from build123d import *

# Parameters (mm, degrees)
F1_DEPTH  = 75
F3_DEPTH  = 4
F5_W      = 61.9195103645
F5_H      = 37.6517623663
F6_DEPTH  = 17
F7_DEPTH  = 44
F9_D      = 7
F9_DEPTH  = 15
F9_TIP    = 2.1030121666
F10_R     = 3.3275648112
F10_R_2   = 1.7
F11_DEPTH = 2
F12_DEPTH = 25.4


with BuildPart() as f1:
    # F0 (on Right) → F1 (new body)
    with BuildSketch(Plane.YZ):
        with BuildLine():
            add(Edge.make_bspline(
                [(-17.7810950981, -27.3124240728), (-18.19174778, -28.0218574236), (-18.6022967338, -28.732065323), (-19.0125334596, -29.4428684699)],
                knots=[0.9798659686, 0.9798659686, 0.9798659686, 0.9798659686, 1, 1, 1, 1], degree=3))
            ThreePointArc((-17.7810950981, -27.3124240728), (-18.4276280065, -28.3598353366), (-19.0125334596, -29.4428684699))
        make_face()
        with BuildLine():
            add(Edge.make_bspline(
                [(21.1806873749, 54.7040760765), (20.2999017837, 46.0225748891), (14.3499977593, 26.8402827287), (-5.7827936538, -6.5844571681), (-17.7810950981, -27.3124240728)],
                knots=[0, 0, 0, 0, 0.3915971259, 0.9798659686, 0.9798659686, 0.9798659686, 0.9798659686], degree=3))
            add(Edge.make_bspline(
                [(-17.7810950981, -27.3124240728), (-18.19174778, -28.0218574236), (-18.6022967338, -28.732065323), (-19.0125334596, -29.4428684699)],
                knots=[0.9798659686, 0.9798659686, 0.9798659686, 0.9798659686, 1, 1, 1, 1], degree=3))
            ThreePointArc((-19.0125334596, -29.4428684699), (-5.934227846, -59.4519469715), (21.1806873749, -41.1116022965))
            Line((21.1806873749, -41.1116022965), (21.1806873749, 54.7040760765))
        make_face()
    extrude(amount=F1_DEPTH)

    # F2 (on face) → F3 (cut)
    with BuildSketch(Plane.YZ.offset(75)):
        with BuildLine():
            Line((5.715811355, -44.2500978365), (17.0802870953, -41.4346371949))
            ThreePointArc((17.0802870953, -41.4346371949), (20.0802870953, -38.4346371949), (17.0802870953, -35.4346371949))
            Line((17.0802870953, -35.4346371949), (5.715811355, -32.6191765533))
            Line((5.715811355, -32.6191765533), (3.0802870953, -21.4346371949))
            ThreePointArc((3.0802870953, -21.4346371949), (0.0802870953, -18.4346371949), (-2.9197129047, -21.4346371949))
            Line((-2.9197129047, -21.4346371949), (-5.5552371643, -32.6191765533))
            Line((-5.5552371643, -32.6191765533), (-16.9197129047, -35.4346371949))
            ThreePointArc((-16.9197129047, -35.4346371949), (-19.9197129047, -38.4346371949), (-16.9197129047, -41.4346371949))
            Line((-16.9197129047, -41.4346371949), (-5.5552371643, -44.2500978365))
            Line((-5.5552371643, -44.2500978365), (-2.9197129047, -55.4346371949))
            ThreePointArc((-2.9197129047, -55.4346371949), (0.0802870953, -58.4346371949), (3.0802870953, -55.4346371949))
            Line((3.0802870953, -55.4346371949), (5.715811355, -44.2500978365))
        make_face()
    extrude(amount=-F3_DEPTH, mode=Mode.SUBTRACT)

    # F5 (on offset) → F6 (cut)
    with BuildSketch(Plane.YZ.offset(50)):
        with Locations((0, -48.4619401395)):
            Rectangle(F5_W, F5_H)
    extrude(amount=F6_DEPTH, mode=Mode.SUBTRACT)

    # F5 (on offset) → F7 (cut)
    with BuildSketch(Plane.YZ.offset(50)):
        with Locations((0, -48.4619401395)):
            Rectangle(F5_W, F5_H)
    extrude(amount=-F7_DEPTH, mode=Mode.SUBTRACT)

    # F9
    with Locations(Plane(origin=(0, 0, 0), x_dir=(0, -1, 0), z_dir=(-1, 0, 0))):
        with Locations((-0.0107965604, -38.4317387827)):
            Hole(F9_D / 2, depth=F9_DEPTH)
            with Locations((0, 0, -(F9_DEPTH + F9_TIP / 2))):  # 118° drill point
                Cone(0, F9_D / 2, F9_TIP, mode=Mode.SUBTRACT)

    # F10 (on face) → F11 (cut)
    with BuildSketch(Plane(origin=(67, 0, 0), x_dir=(0, -1, 0), z_dir=(-1, 0, 0))):
        with Locations((0, -38.3945740759)):
            Circle(F10_R)
        with Locations((0, -38.3945740759)):
            Circle(F10_R_2, mode=Mode.SUBTRACT)
    extrude(amount=-F11_DEPTH, mode=Mode.SUBTRACT)

    # F10 (on face) → F12 (cut)
    with BuildSketch(Plane(origin=(67, 0, 0), x_dir=(0, -1, 0), z_dir=(-1, 0, 0))):
        with Locations((0, -38.3945740759)):
            Circle(F10_R_2)
    extrude(amount=-F12_DEPTH, mode=Mode.SUBTRACT)


solid = f1.part
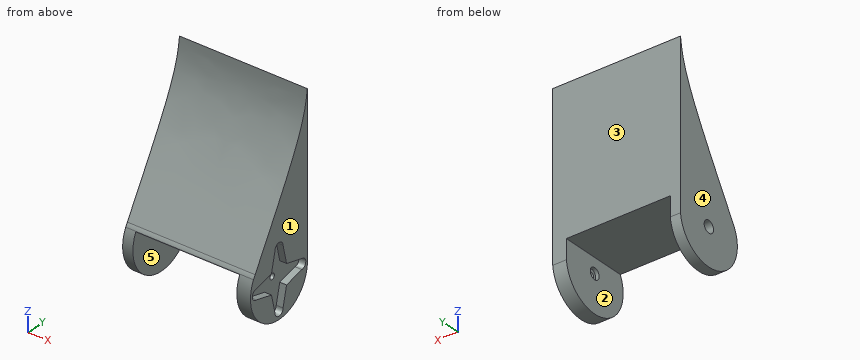
Read the model definition and answer for the solid it produces. Units are mm, in the model's axes. Face numbers are marked on the shaded views. A direction names the side the tool comes from. Round coordinates to 2 decimals unless told otherwise and drop trailing zeros. One line per question, with ' | ' between items. Start each with the question number.
1. Find the intervals of material crossed by probe 1 along X at (y, z) = (-5, -41.5); probe 2 along X at (y, z) = (7, -31); probe 3 along Y at (x, z) = (5, -39), in increasing order. Write a range as [from, to].
2. For a pull along X with two mould halves and no side action, classify the marked faces 1, 2 and 3 as +X half, -X half, draft (parallel to the pull), parting line (faces both ways), or undercut.
3. Each of these flat-tipped pins is pushed along its axis until it touches: pin 1 (5 mm diameter, centred on y = 10.5, z = 33, fed in from -X); pin 2 (12 mm diameter, centred on x = 36, z = 41.5, fed in from -Y); pin 3 (7.5 mm diameter, centred on y = 1, z = -39, fed in from -X); pin 4 (7.5 mm diameter, centred on y = 0, z = -38.39, fed in from +X). Where does it stop, or does it pass through?
4. Section A-A (y = 0) is taken. Give the number of separate pieces and of enclosed holes in the cut face, and give its area (3 significant figures).
5. For the marked faces 4 and 5, determine the directions among +Z, -Z, +X, -X, +Y, -Y from which every point of the face is accessible in a straight line to the end or side of a thin tool.
Filled in:
1) probe 1: [0, 6], [67, 71] | probe 2: [0, 6], [67, 75] | probe 3: [-21.28, -3.44], [3.46, 21.18]
2) face 1: +X half | face 2: undercut | face 3: draft
3) pin 1: through | pin 2: y = 16.35 | pin 3: x = 0 | pin 4: x = 71
4) separate pieces: 3 | enclosed holes: 0 | area: 2,680 mm²
5) face 4: +Z, -Z, -X, +Y, -Y | face 5: -Z, +Y, -Y
